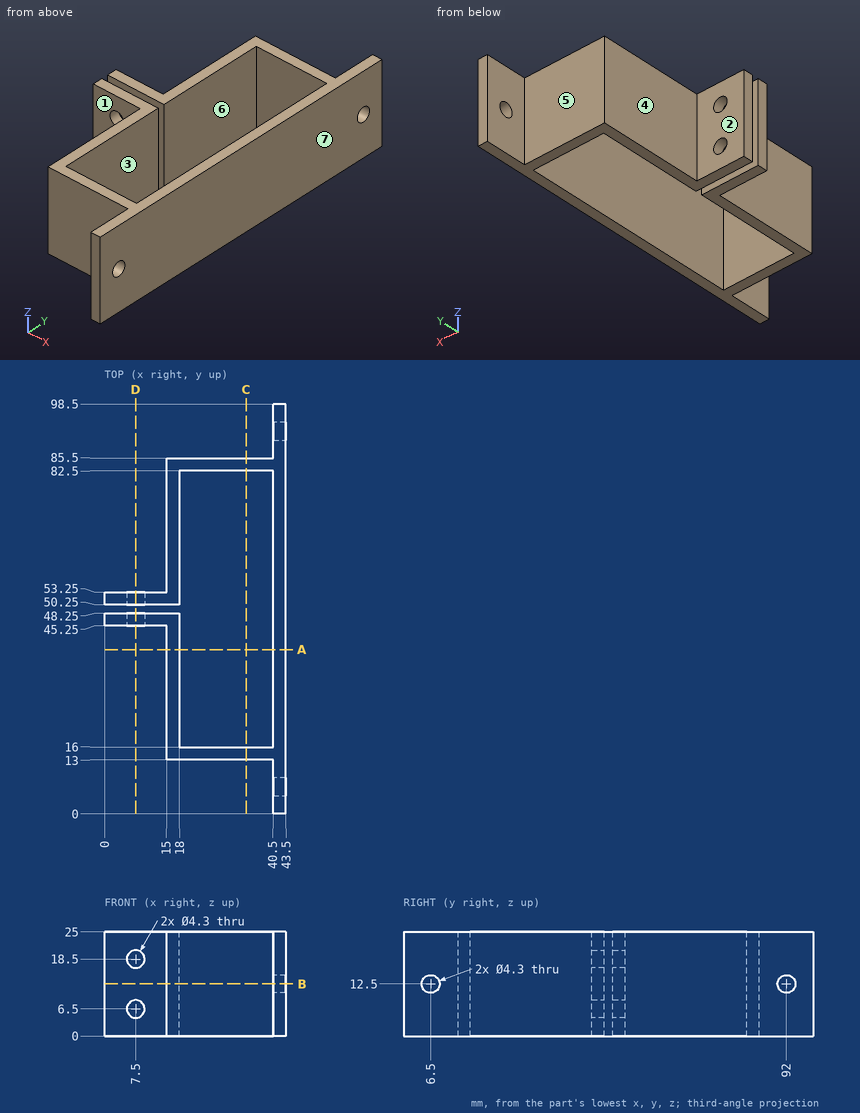
Part print with two shaded views. Sizes in mm from the minimum x, y, z corner. A direction names the side the tool comes from. Coordinates: 2 decimals unless noted, no trailing zeros. Write each loop counter-clockwise with the first axis right and the second up, starting at its lowest first coordinate (ties: lowest second). Pieces come first, ordered by that corner, then holes.
(1) Drill centre lines: line 1 (X direction, y = 46.2, z = 6.5); line 2 (Y direction, x = 32, z = 9.5); line 3 (Z direction, x = 7.5, y = 46.45). Where is each one in solid material? Low to high.
(2) Pin check, flat tips, straight feed: pin 1 Ø5.5 at (x, z) = (6.5, 12) entering from -Y; pin 2 Ø7.5 at (y, z) = (62, 11.5) entering from -X; pin 3 Ø7 at (x, z) = (24, 12) entering from -Y. Stop position of each tip, or through.
(3) Cut at A-A on y = 39.5. List the corners of the cut face in (x, z), and give its area (3 significant figures).
(4) 3-axis set-ups, long thin cutter, end or side, ignore diameter. For the marked faces 1, 2 and 3: which of +Z, -Z, +X, -X, +Y, -Y reach the whole face in a straight line?
(5) Cut at C-C on x = 34. List the corners of the cut face in (y, z), and give its area (3 significant figures).
(6) Cut at D-D on x = 7.5. List the corners of the cut face in (y, z), and give its area (3 significant figures).
(7) Mould opens along X. For the marked faces 4, 5, 6 and 7 say: pulls with the +X half, pulls with the -X half, needs draft (parallel to the pull), parting line crosses it, or undercut.
(8) Cut at B-B on z = 12.5. List the corners of the cut face in (x, y).
Working result:
1. line 1: x = 0 to 5.35, 9.65 to 18, 40.5 to 43.5
1. line 2: y = 13 to 16, 82.5 to 85.5
1. line 3: z = 0 to 4.35, 8.65 to 16.35, 20.65 to 25
2. pin 1: stops at y = 45.25
2. pin 2: stops at x = 15
2. pin 3: stops at y = 13
3. outline: (15, 0) - (18, 0) - (18, 25) - (15, 25) - close; (40.5, 0) - (43.5, 0) - (43.5, 25) - (40.5, 25) - close
3. area: 150 mm2
4. face 1: +Z, -Z, -X, -Y
4. face 2: +Z, -Z, -X, +Y
4. face 3: +Z, -Z
5. outline: (13, 0) - (16, 0) - (16, 25) - (13, 25) - close; (82.5, 0) - (85.5, 0) - (85.5, 25) - (82.5, 25) - close
5. area: 150 mm2
6. outline: (45.25, 0) - (48.25, 0) - (48.25, 4.35) - (45.25, 4.35) - close; (45.25, 8.65) - (48.25, 8.65) - (48.25, 16.35) - (45.25, 16.35) - close; (45.25, 20.65) - (48.25, 20.65) - (48.25, 25) - (45.25, 25) - close; (50.25, 0) - (53.25, 0) - (53.25, 4.35) - (50.25, 4.35) - close; (50.25, 8.65) - (53.25, 8.65) - (53.25, 16.35) - (50.25, 16.35) - close; (50.25, 20.65) - (53.25, 20.65) - (53.25, 25) - (50.25, 25) - close
6. area: 98.4 mm2
7. face 4: pulls with the -X half
7. face 5: needs draft
7. face 6: undercut
7. face 7: pulls with the +X half
8. outline: (0, 45.25) - (15, 45.25) - (15, 13) - (40.5, 13) - (40.5, 8.65) - (43.5, 8.65) - (43.5, 89.85) - (40.5, 89.85) - (40.5, 85.5) - (15, 85.5) - (15, 53.25) - (0, 53.25) - (0, 50.25) - (18, 50.25) - (18, 82.5) - (40.5, 82.5) - (40.5, 16) - (18, 16) - (18, 48.25) - (0, 48.25) - close; (40.5, 0) - (43.5, 0) - (43.5, 4.35) - (40.5, 4.35) - close; (40.5, 94.15) - (43.5, 94.15) - (43.5, 98.5) - (40.5, 98.5) - close
